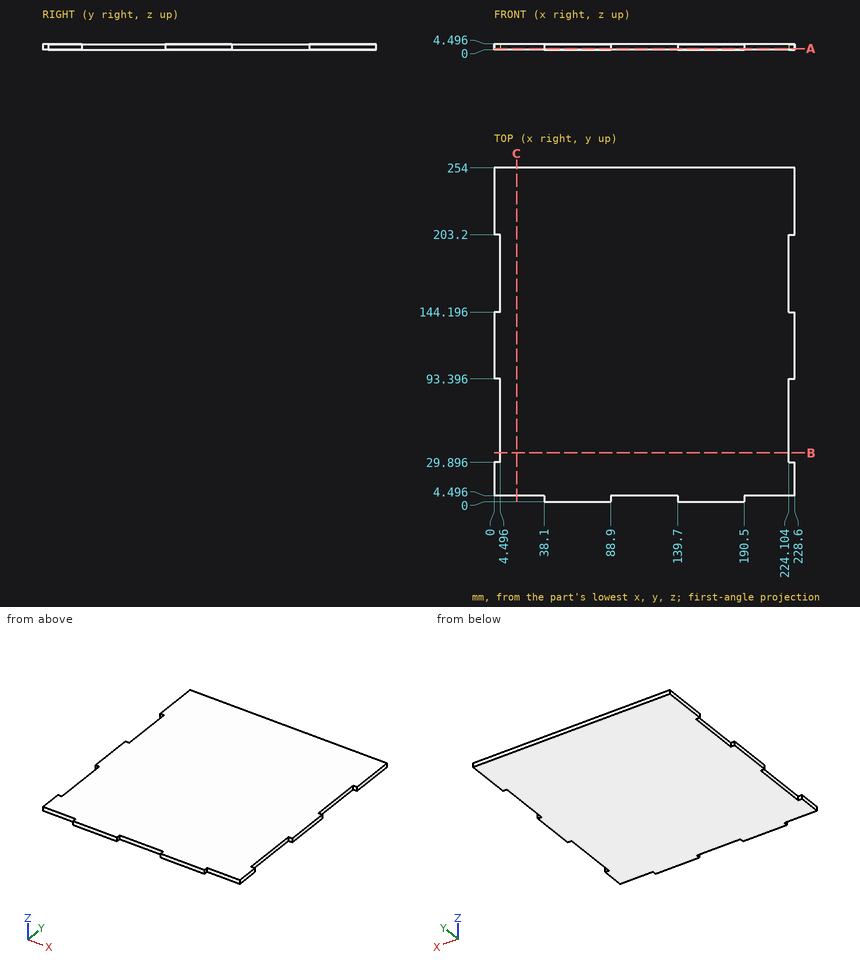
Design review of the part shown in the three views and the two pictorial views. Dimensions are in mm from the part's minimum x, y and z. Round coordinates to 2 decimals unless told otherwise and drop trailing zeros. Write each loop counter-clockwise with the first axis right and the second up, starting at its lowest first coordinate (ties: lowest second). Pieces come first, ordered by that corner, then holes.
Item 1: We need section A-A on z = 1.05. Write out the cut boundary in (x, y).
Item 2: For probe 1 along Y at (x, z) = (199, 3.7); probe 2 along X at (y, z) = (179, 0.2), list the stretches that pass through material, from the lowest coordinate up.
Item 3: We need section B-B on y = 37. Write out the cut boundary in (x, z).
Item 4: Clearance check with flat-ended pins moving along their axes: pin 1 Ø1.3 at (x, z) = (126.5, 3) entering from -Y; pin 2 Ø2 at (y, z) = (3, 2.5) entering from -X; pin 3 Ø2 at (y, z) = (3, 3.5) entering from +X. State where each tip first meets the part, or that it passes through.
Item 5: We need section C-C on x = 17. Write out the cut boundary in (y, z), and give its area (3 significant figures).
Returned:
1. outline: (0, 4.5) - (38.1, 4.5) - (38.1, 0) - (88.9, 0) - (88.9, 4.5) - (139.7, 4.5) - (139.7, 0) - (190.5, 0) - (190.5, 4.5) - (228.6, 4.5) - (228.6, 29.9) - (224.1, 29.9) - (224.1, 93.4) - (228.6, 93.4) - (228.6, 144.2) - (224.1, 144.2) - (224.1, 203.2) - (228.6, 203.2) - (228.6, 254) - (0, 254) - (0, 203.2) - (4.5, 203.2) - (4.5, 144.2) - (0, 144.2) - (0, 93.4) - (4.5, 93.4) - (4.5, 29.9) - (0, 29.9) - close
2. probe 1: y = 4.5 to 254
2. probe 2: x = 4.5 to 224.1
3. outline: (4.5, 0) - (224.1, 0) - (224.1, 4.5) - (4.5, 4.5) - close
4. pin 1: stops at y = 4.5
4. pin 2: stops at x = 38.1
4. pin 3: stops at x = 190.5
5. outline: (4.5, 0) - (254, 0) - (254, 4.5) - (4.5, 4.5) - close
5. area: 1,120 mm2
